Study the drawing (mm; zero at the part's minimum x, y, z) and answer. A direction names the side the tool comes from. Round coordinates to 2 decimals unless told otherwise and drop trailing zeros. Write each loop counter-clockwise with the first axis right and the second up, starting at its lowest first coordinate (ties: lowest second). Pieces come first, ordered by that corner, then holes. Notation, with made-up numbers: (79, -9) - (95, -9) arc R22 cw to (95, 19) - close; hole circle Ø4 at (-34.5, 23.5). An arc over 180 degrees is marked (long way). Return JSON: item names as keys, results as strings. Group by question number.
(1) Section A-A, the plane x = 42.5 is taken. Write down the section's boundary in (y, z).
(2) Each of these flat-tipped pins is pushed along its axis until it touches: pin 1 (1 mm diameter, centred on y = 34.5, z = 20.5, fed in from +X); pin 2 (3 mm diameter, centred on y = 70.5, z = 21.5, fed in from -X); pin 3 (2 mm diameter, centred on y = 60, z = 15, fed in from -X). Where does it stop, or does it pass through?
(3) Which of the six approach directions +Z, -Z, +X, -X, +Y, -Y give full straight-line access (tool end or side, diameter ignored) to the marked faces 1 and 2?
(4) Section C-C, the plane z = 16.5 is taken. Write down the section's boundary in (x, y), then the cut area to 3 significant figures.
(5) Section B-B, the plane y = 42.5 is taken. Write down the section's boundary in (x, z), then the cut area to 4 significant figures.
(6) Find the intervals of material crossed by line 1 along Y through (x, z) = (42.5, 22.85); line 2 along Y through (x, z) = (42.5, 11.5); line 3 along X through (y, z) = (58.5, 20.5), in increasing order. Write a range as [from, to].
(7) Determine the mould class of the marked faces 3, 4 and 5 for opening direction Y: +Y half, -Y half, draft (parallel to the pull), parting line (faces both ways), or undercut.
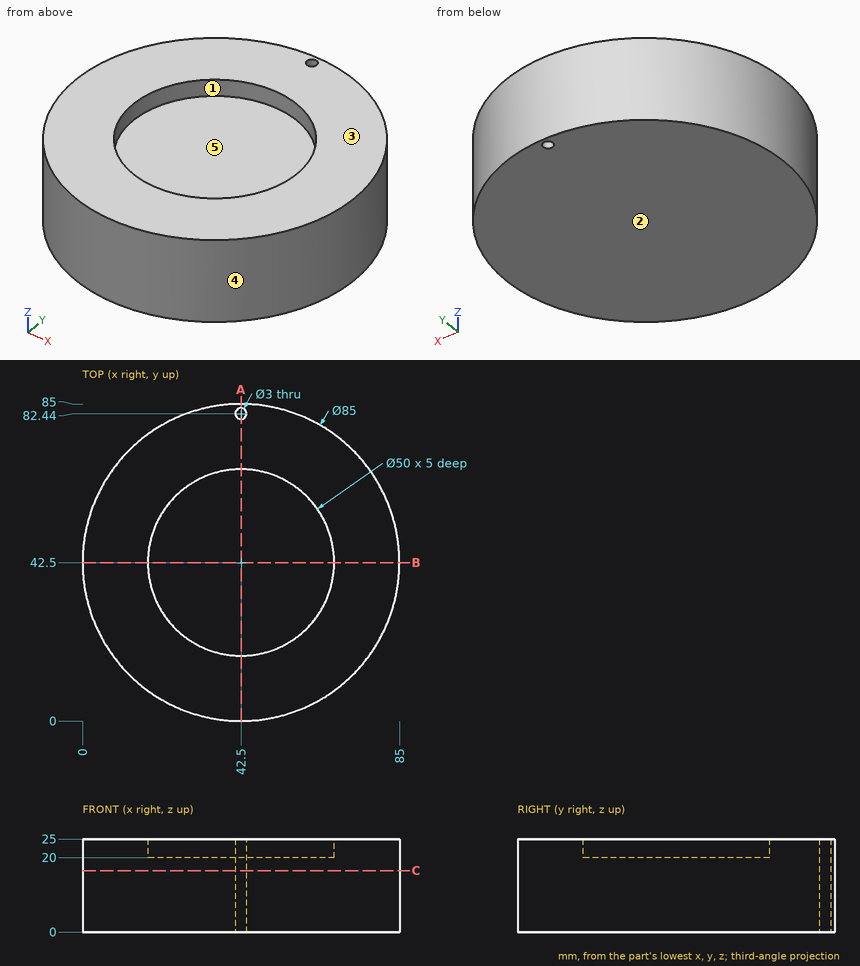
Working result:
{
 "1": {"outline": "(0, 0) - (80.94, 0) - (80.94, 25) - (67.5, 25) - (67.5, 20) - (17.5, 20) - (17.5, 25) - (0, 25) - close; (83.94, 0) - (85, 0) - (85, 25) - (83.94, 25) - close"},
 "2": {"pin 1": "stops at x = 84.33", "pin 2": "stops at x = 9.27", "pin 3": "stops at x = 3.33"},
 "3": {"face 1": "+Z", "face 2": "-Z, +X, -X, +Y, -Y"},
 "4": {"outline": "circle Ø85 at (42.5, 42.5); hole circle Ø3 at (42.5, 82.44)", "area": "5,670 mm^2"},
 "5": {"outline": "(0, 0) - (85, 0) - (85, 25) - (67.5, 25) - (67.5, 20) - (17.5, 20) - (17.5, 25) - (0, 25) - close", "area": "1,875 mm^2"},
 "6": {"line 1": "y = [0, 17.5], [67.5, 80.94], [83.94, 85]", "line 2": "y = [0, 80.94], [83.94, 85]", "line 3": "x = [3.13, 23.29], [61.71, 81.87]"},
 "7": {"face 3": "draft", "face 4": "parting line", "face 5": "undercut"}
}
